Here's how the part is built. I have some questions about the finished solid (model axes, mm). Coordinates: 2 decimals unless noted, no trailing zeros. Write each loop counter-clockwise with the first axis right and the second up, starting at its lowest first coordinate (ties: lowest second). Pieces come first, ordered by that corner, then holes.
```python
from build123d import *

# Parameters (mm, degrees)
SKETCH1_R           = 2.725
SKETCH1_R_2         = 1.575
BOSS_EXTRUDE1_DEPTH = 3
DEBURS_SIZE         = 0.2


with BuildPart() as part:
    # Sketch1 → Boss-Extrude1 (new body)
    with BuildSketch(Plane.XY):
        Circle(SKETCH1_R)
        Circle(SKETCH1_R_2, mode=Mode.SUBTRACT)
    extrude(amount=BOSS_EXTRUDE1_DEPTH)

    # Deburs
    deburs_edges = [part.edges().sort_by_distance(p)[0] for p in [
        (-2.725, 0, 0),
        (-2.725, 0, 3),
        (-1.575, 0, 0),
        (-1.575, 0, 3),
    ]]
    chamfer(deburs_edges, length=DEBURS_SIZE)


solid = part.part
```
1) Will these pins go through, and if not, where does the flat tip stop? pin 1 (3 mm diameter, centred on x = 0, y = 0, fed in from +Z); pin 2 (1.5 mm diameter, centred on x = 2, z = 1, fed in from +Y); pin 3 (1 mm diameter, centred on y = 1.5, z = 1, fed in from +X).
Values follow:
pin 1: passes through
pin 2: stops at y = 2.42
pin 3: stops at x = 2.53
2) Imagine slicing it at A-A on y = 0. Please give me the cut outline in (x, z) (3 decimals), then the cut area to 3 significant figures.
Values follow:
outline: (-2.725, 0.2) - (-2.525, 0) - (-1.775, 0) - (-1.575, 0.2) - (-1.575, 2.8) - (-1.775, 3) - (-2.525, 3) - (-2.725, 2.8) - close; (1.575, 0.2) - (1.775, 0) - (2.525, 0) - (2.725, 0.2) - (2.725, 2.8) - (2.525, 3) - (1.775, 3) - (1.575, 2.8) - close
area: 6.74 mm2
3) We'd pull the mould along Y, two halves only. Please class faces 1 (the face through (-1.25, -0.96, 1.48)), 2 (the face through (1, 2, 3)), 3 (the face through (2.6, 0.82, 1.48)): pulls with the +Y half, pulls with the -Y half, needs draft (parallel to the pull), parting line crosses it, or undercut.
Values follow:
face 1: undercut
face 2: needs draft
face 3: parting line crosses it
4) Imagine slicing it at C-C on z = 0.5. Please give me the cut outline in (x, y) (3 decimals), then the cut area to 3 significant figures.
Values follow:
outline: circle Ø5.45 at (0, 0); hole circle Ø3.15 at (0, 0)
area: 15.5 mm2
5) I need wall thicknesses on probe 1 along Y at (x, z) = (0, 2) (3 decimals); probe 2 along Y at (x, z) = (0.85, 2.35); probe 3 along X at (y, z) = (-0.35, 2.4). Which ranges of each line are inside material? Lowest first, please.
Values follow:
probe 1: y = -2.725 to -1.575, 1.575 to 2.725
probe 2: y = -2.59 to -1.33, 1.33 to 2.59
probe 3: x = -2.7 to -1.54, 1.54 to 2.7
